Source: CAD feature listing. Evaluate the final solid. Frame: model axes, mm. A direction names the side the tool comes from. Give positions to 0.01 mm unless a question says otherwise; leave off trailing zeros. Order: outer loops, then holes, each group sorted by start corner. A loop starts at its lowest first (then second) coordinate and runs counter-clockwise, first axis right, second up.
from build123d import *

# Parameters (mm, degrees)
SKETCH3_W                  = 63.5
SKETCH3_H                  = 9.525
BOSS_EXTRUDE1_DEPTH        = 12.7
TAP_DRILL_FOR_10_24_TAP1_D = 3.7973
SKETCH11_W                 = 12.7
SKETCH11_H                 = 6.35
BOSS_EXTRUDE2_DEPTH        = 25.4
F_8_CLEARANCE_HOLE2_D      = 4.4958
FILLET1_R                  = 6.35


with BuildPart() as part:
    # Sketch3 → Boss-Extrude1 (new body)
    with BuildSketch(Plane.XY):
        with Locations((31.75, 4.7625)):
            Rectangle(SKETCH3_W, SKETCH3_H)
    extrude(amount=BOSS_EXTRUDE1_DEPTH)

    # Tap Drill for #10-24 Tap1 (through all)
    with Locations(Plane(origin=(0, 9.525, 0), x_dir=(1, 0, 0), z_dir=(0, 1, 0))):
        with Locations((57.15, -4.7625), (6.35, -4.7625), (31.75, -4.7625)):
            Hole(TAP_DRILL_FOR_10_24_TAP1_D / 2)

    # Sketch11 → Boss-Extrude2 (add)
    with BuildSketch(Plane.XY.offset(12.7)):
        with Locations((6.35, 6.35)):
            Rectangle(SKETCH11_W, SKETCH11_H)
        with Locations((57.15, 6.35)):
            Rectangle(SKETCH11_W, SKETCH11_H)
    extrude(amount=BOSS_EXTRUDE2_DEPTH)

    # #8 Clearance Hole2 (through all)
    with Locations(Plane.ZY):
        with Locations((30.1625, 6.35)):
            Hole(F_8_CLEARANCE_HOLE2_D / 2)

    # Fillet1
    fillet1_edges = [part.edges().sort_by_distance(p)[0] for p in [
        (12.7, 6.35, 12.7),
        (50.8, 6.35, 12.7),
    ]]
    fillet(fillet1_edges, radius=FILLET1_R)


solid = part.part
1) Ray query, L1, parallel to X at y = 2.75, z = 5; L2, parallel to Z at x = 31.75, y = 7; L3, parallel to X at y = 6.75, z = 24.5. Return the intervals inside material, ascending.
Checks:
L1: x = 0 to 4.47, 8.23 to 29.87, 33.63 to 55.27, 59.03 to 63.5
L2: z = 0 to 2.86, 6.66 to 12.7
L3: x = 0 to 12.7, 50.8 to 63.5
2) Pull-direction query (Z, two-part tool) for faces 1 (the face through (56, 3.175, 25)), 2 (the face through (7.857, 4.696, 5.918)), 3 (the face through (57, 6, 38.1)); classes: +Z half, -Z half, draft (parallel to the pull), parting line (faces both ways), or undercut.
Checks:
face 1: draft
face 2: undercut
face 3: +Z half
3) Section query C-C on y = 5.5. Output: boundary loops of the cut face in (x, z).
Checks:
outline: (0, 0) - (63.5, 0) - (63.5, 28.08) - (50.8, 28.08) - (50.8, 19.05) arc R6.35 cw to (44.45, 12.7) - (19.05, 12.7) arc R6.35 cw to (12.7, 19.05) - (12.7, 28.08) - (0, 28.08) - close; (0, 32.24) - (12.7, 32.24) - (12.7, 38.1) - (0, 38.1) - close; (50.8, 32.24) - (63.5, 32.24) - (63.5, 38.1) - (50.8, 38.1) - close; hole circle Ø3.8 at (6.35, 4.76); hole circle Ø3.8 at (31.75, 4.76); hole circle Ø3.8 at (57.15, 4.76)
4) First-contact query: pin 1 Ø5 at (x, y) = (24, 6.5) entering from +Z; pin 2 Ø5.5 at (x, z) = (49.5, 21.5) entering from -Y (3 decimals). Flat tips, straight axial feed; report the tip coordinate or a pass-through.
Checks:
pin 1: stops at z = 12.7
pin 2: stops at y = 3.175
5) Section query D-D on z = 13.5. Output: boundary loops of the cut face in (x, y) (3 decimals).
Checks:
outline: (0, 3.175) - (15.965, 3.175) - (15.965, 9.525) - (0, 9.525) - close; (47.535, 3.175) - (63.5, 3.175) - (63.5, 9.525) - (47.535, 9.525) - close
6) Reachability of faces 4 (the face through (31, 4, 12.7)), 5 (the face through (30, 4.7, 5.5)), 6 (the face through (31, 5, 0)), 7 (the face through (7, 3.175, 25)), 8 (the face through (14.61, 6.39, 14.51)) from +Z, -Z, +X, -X, +Y, -Y: full face, straight path, thin tool, end or side. Return the list, or none.
Checks:
face 4: +Z, -Y
face 5: +Y, -Y
face 6: -Z, +X, -X, +Y, -Y
face 7: +Z, +X, -X, -Y
face 8: +Z, +Y, -Y
7) Section query A-A on x = 31.75. Output: boundary loops of the cut face in (y, z) (3 decimals), and give its area (3 significant figures).
Checks:
outline: (0, 0) - (9.525, 0) - (9.525, 2.864) - (0, 2.864) - close; (0, 6.661) - (9.525, 6.661) - (9.525, 12.7) - (0, 12.7) - close
area: 84.8 mm2
8) Section query B-B on x = 6.35. State how many separate pieces and enclosed holes the cut face has, and give its area (3 significant figures).
Checks:
separate pieces: 2
enclosed holes: 1
area: 230 mm2
